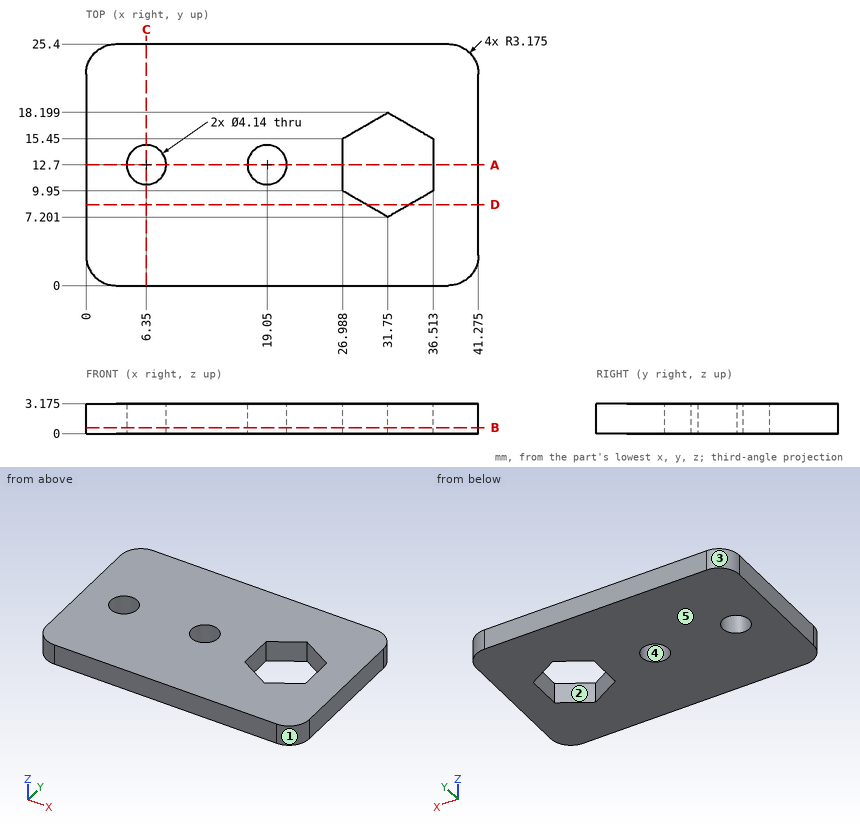
Geometry: see drawing. Coordinates: mm, zero at the bounding-box minimum. A direction names the side the tool comes from. Coordinates: 2 decimals unless noted, no trailing zeros. Loops run counter-clockwise (first coordinate to the right, second up) from the corner with the lowest first, then second, coordinate; pieces in that order, holes last.
(1) Section B-B on z = 0.65. Count the separate pieces of the cut face and the enclosed holes in it, then the cut area to 3 significant figures.
(2) Material intervals for probe 1 along Y at (x, z) = (19.05, 1.9); probe 2 along X at (y, z) = (10, 2.3) (1 decimal); probe 3 along X at (y, z) = (13.75, 3) (1 decimal), sorted ascending.
(3) Section C-C on x = 6.35. Return the cut outline in (y, z) (1 decimal).
(4) First-contact query: pin 1 Ø3.5 at (x, y) = (19.05, 12.7) entering from -Z. Flat tip, straight axial feed; report the tip coordinate or a pass-through.
(5) Pull-direction query (Y, two-part tool) for the marked faces 3, 4 and 5; classes: released by +Y, released by -Y, zero draft, split by the parting line, or undercut.
(6) Section A-A on y = 12.7. Return the cut outline in (x, z) (1 decimal).
(7) Section D-D on y = 8.5. Return the cut outline in (x, z) (1 decimal).
(8) Set-up query: the marked faces 1 and 2. Return all of +Z, -Z, +X, -X, +Y, -Y with unobstructed straight access to the full face (end or side cutting, diameter ignored); none if empty.
Data:
1. separate pieces: 1
1. enclosed holes: 3
1. area: 934 mm2
2. probe 1: y = 0 to 10.63, 14.77 to 25.4
2. probe 2: x = 0 to 27, 36.5 to 41.3
2. probe 3: x = 0 to 4.6, 8.1 to 17.3, 20.8 to 27, 36.5 to 41.3
3. outline: (0, 0) - (10.6, 0) - (10.6, 3.2) - (0, 3.2) - close; (14.8, 0) - (25.4, 0) - (25.4, 3.2) - (14.8, 3.2) - close
4. pin 1: passes through
5. face 3: released by +Y
5. face 4: undercut
5. face 5: zero draft
6. outline: (0, 0) - (4.3, 0) - (4.3, 3.2) - (0, 3.2) - close; (8.4, 0) - (17, 0) - (17, 3.2) - (8.4, 3.2) - close; (21.1, 0) - (27, 0) - (27, 3.2) - (21.1, 3.2) - close; (36.5, 0) - (41.3, 0) - (41.3, 3.2) - (36.5, 3.2) - close
7. outline: (0, 0) - (29.5, 0) - (29.5, 3.2) - (0, 3.2) - close; (34, 0) - (41.3, 0) - (41.3, 3.2) - (34, 3.2) - close
8. face 1: +Z, -Z, +X, -Y
8. face 2: +Z, -Z
